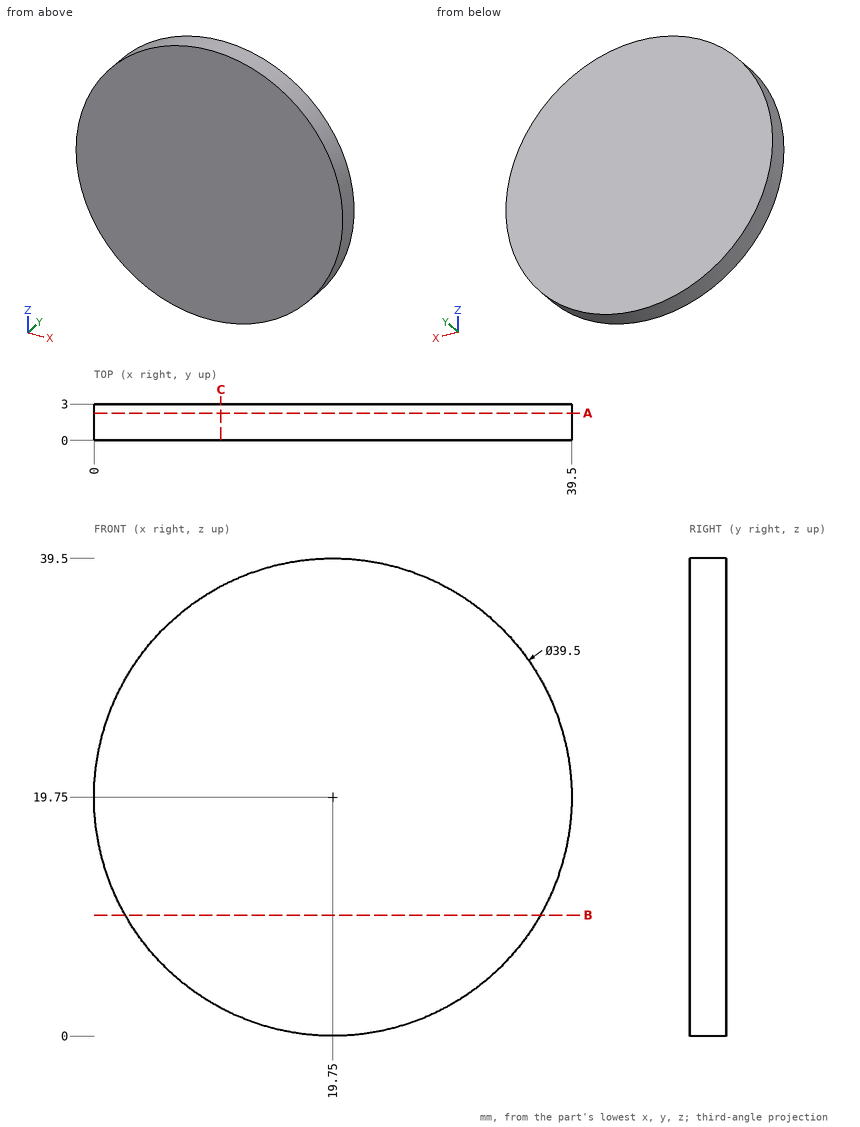
For this review, use the dimensioned drawing (mm, ordinates from the lowest corner) and the shaded views. Coordinates: 2 decimals unless noted, no trailing zeros. Loops run counter-clockwise (first coordinate to the right, second up) from the corner with the lowest first, then second, coordinate; pieces in that order, holes last. Notation, with made-up numbers: (-8, 41.25) -> (48, 41.25) arc R6 cw to (48, 46.25) -> close; hole circle Ø9 at (52.25, 43). An arc over 180 degrees is marked (long way). Use a Markdown table: item, result. Add a question column.
Item 1: We need section A-A, the plane y = 2.25. Write out the cut boundary in (x, z).
Item 2: We need section C-C, the plane x = 10.5. Write out the cut boundary in (y, z), and give its area (3 significant figures).
Item 3: We need section B-B, the plane z = 10. Write out the cut boundary in (x, y), and give its area (3 significant figures).
Item 4: Wall thickness on L1, parallel to X at y = 2.3, z = 20; L2, parallel to Z at x = 26.5, y = 1.45; L3, parallel to X at y = 1, z = 37: over which ranges is each line inside the solid? List them lowest first. Write a range as from..to.
Numbers:
| question | item | result |
|---|---|---|
| 1 | outline | circle Ø39.5 at (19.75, 19.75) |
| 2 | outline | (0, 2.3) -> (3, 2.3) -> (3, 37.2) -> (0, 37.2) -> close |
| 2 | area | 105 mm^2 |
| 3 | outline | (2.57, 0) -> (36.93, 0) -> (36.93, 3) -> (2.57, 3) -> close |
| 3 | area | 103 mm^2 |
| 4 | L1 | x = 0..39.5 |
| 4 | L2 | z = 1.19..38.31 |
| 4 | L3 | x = 10.13..29.37 |
